```python
from build123d import *
from build123d.topology import SkipClean

# Parameters (mm, degrees)
SKETCH2_R               = 120
BOSS_EXTRUDE2_DEPTH     = 85
SKETCH3_R               = 116
CUT_EXTRUDE1_DEPTH      = 82
CUT_EXTRUDE5_DEPTH      = 2
CUT_EXTRUDE5_DEPTH_BACK = 2
SKETCH8_R               = 75
SKETCH9_R               = 32
CUT_EXTRUDE6_DEPTH      = 5
BOSS_EXTRUDE4_START     = 40
SKETCH12_R              = 32
BOSS_EXTRUDE4_DEPTH     = 40


with BuildPart() as part:
    # Sketch2 → Boss-Extrude2 (new body)
    with BuildSketch(Plane.XY):
        Circle(SKETCH2_R)
    extrude(amount=BOSS_EXTRUDE2_DEPTH)

    # Sketch3 → Cut-Extrude1 (cut)
    with BuildSketch(Plane.XY.offset(85)):
        Circle(SKETCH3_R)
    extrude(amount=-CUT_EXTRUDE1_DEPTH, mode=Mode.SUBTRACT)

    # Sketch8 → Cut-Extrude5 (cut, two sides: drawn at the far end of the back side and taken through both)
    with BuildSketch(Plane.XY.offset(3).offset(-CUT_EXTRUDE5_DEPTH_BACK)):
        Circle(SKETCH8_R)
    extrude(amount=CUT_EXTRUDE5_DEPTH + CUT_EXTRUDE5_DEPTH_BACK, mode=Mode.SUBTRACT)

    # Sketch9 → Cut-Extrude6 (cut)
    with BuildSketch(Plane.XY.offset(1)):
        Circle(SKETCH9_R)
    extrude(amount=-CUT_EXTRUDE6_DEPTH, mode=Mode.SUBTRACT)

    # Sketch12 → Boss-Extrude4 (add)
    # profile 1 of 2: a face of its own
    with SkipClean():  # the faces are left unmerged after this step: merging them gives an invalid solid
        with BuildSketch(Plane(origin=(0, 0, 0), x_dir=(-1, 0, 0), z_dir=(0, 0, -1)).offset(BOSS_EXTRUDE4_START)):
            with BuildLine():
                ThreePointArc((120, 0), (0, 120), (-120, 0))
                Line((-120, 0), (-118.831087629, -16.70845932))
                ThreePointArc((-118.831087629, -16.70845932), (-3.111785776, -119.959646504), (117.805011812, -22.84686394))
                Line((117.805011812, -22.84686394), (120, 0))
            make_face()
            with Locations(Location((0, 0, 0), (0, 0, 180))):
                Circle(SKETCH12_R, mode=Mode.SUBTRACT)
        # profile 2 of 2: a face of its own
        with BuildSketch(Plane(origin=(0, 0, 0), x_dir=(-1, 0, 0), z_dir=(0, 0, -1)).offset(BOSS_EXTRUDE4_START)):
            with BuildLine():
                ThreePointArc((117.805011812, -22.84686394), (-3.111785776, -119.959646504), (-118.831087629, -16.70845932))
                Line((-118.831087629, -16.70845932), (-99.063378042, -299.268538041))
                ThreePointArc((-99.063378042, -299.268538041), (-3.575656086, -388.008129656), (91.309922092, -298.624981255))
                Line((91.309922092, -298.624981255), (117.805011812, -22.84686394))
            make_face()
        extrude(amount=-BOSS_EXTRUDE4_DEPTH)


solid = part.part
```
The listing builds one solid part. Answer for the finished solid, in the listing's coordinates (mm). A direction names the side the tool comes from. Give positions to 0.01 mm unless a question says otherwise; leave off trailing zeros. Loops run counter-clockwise (first coordinate to the right, second up) from the corner with the lowest first, then second, coordinate; pieces in that order, holes last. Notation, with made-up numbers: (77.5, -6) - (120.5, -6) arc R21 ccw to (120.5, 25) - close; hole circle Ø7 at (53, 6.5). An arc over 180 degrees is marked (long way). Answer as CSV lines item,"result". Start each with the question number.
Item 1: A cutting plane is placed at A-A on x = -1. Determine the outline of the cut face in (y, z), then the cut area to 3 significant figures.
Item 2: A cutting plane is placed at C-C on x = -60.5. Determine the outline of the cut face in (y, z).
Item 3: For faces 4 (the face through (-63, 98, 85)), 5 (the face through (-2, -76, 3)), determine the directions among +Z, -Z, +X, -X, +Y, -Y from which every point of the face is accessible in a straight line to the end or side of a thin tool.
Item 4: A cutting plane is placed at B-B on y = -64. Determine the outline of the cut face in (x, z), then the cut area to 3 significant figures.
Item 5: Each of these flat-tipped pins is pushed along its axis until it touches: pin 1 (3 mm diameter, centred on x = -74.5, z = 38.5, fed in from -Y); pin 2 (2 mm diameter, centred on x = 5.5, z = -2.5, fed in from +Y); pin 3 (10 mm diameter, centred on y = -244.5, z = 0.5, fed in from +X). Where does it stop, or does it pass through?
Item 6: A cutting plane is placed at D-D on z = 73. Determine the outline of the cut face in (x, y), then the cut area to 3 significant figures.
Item 7: Find the intervals of material crossed by line 1 (Y direction, x = 0, z = -21); line 2 (Z direction, x = -105, y = -45); line 3 (Z direction, x = -11, y = -277), in increasing order. Write a range as from..to.
Item 8: The mould has two halves that part along X. Classify faces 1 (the face through (2, -241, 0)), 2 (the face through (5.585, -387.994, -20.28)), 3 (the face through (-9.764, 74.362, 1.986)): +X half, -X half, draft (parallel to the pull), parting line (faces both ways), or undercut.
Found:
1,outline,"(-387.88, -40) - (-31.98, -40) - (-31.98, 1) - (-74.99, 1) - (-74.99, 3) - (-116, 3) - (-116, 85) - (-120, 85) - (-120, 0) - (-387.88, 0) - close; (31.98, -40) - (120, -40) - (120, 85) - (116, 85) - (116, 3) - (74.99, 3) - (74.99, 1) - (31.98, 1) - close"
1,area,"18,800 mm^2"
2,outline,"(-362.99, -40) - (103.63, -40) - (103.63, 85) - (98.97, 85) - (98.97, 3) - (44.33, 3) - (44.33, 1) - (-44.33, 1) - (-44.33, 3) - (-98.97, 3) - (-98.97, 85) - (-103.63, 85) - (-103.63, 0) - (-362.99, 0) - close"
3,face 4,"+Z, +X, -X, +Y, -Y"
3,face 5,"+Z"
4,outline,"(-113.85, -40) - (115.52, -40) - (115.52, 0) - (101.51, 0) - (101.51, 85) - (96.75, 85) - (96.75, 3) - (39.1, 3) - (39.1, 1) - (-39.1, 1) - (-39.1, 3) - (-96.75, 3) - (-96.75, 85) - (-101.51, 85) - (-101.51, 0) - (-113.85, 0) - close"
4,area,"10,400 mm^2"
5,pin 1,"stops at y = -95.24"
5,pin 2,"stops at y = 119.92"
5,pin 3,"stops at x = 103.24"
6,outline,"circle Ø240 at (0, 0); hole circle Ø232 at (0, 0)"
6,area,"2,970 mm^2"
7,line 1,"y = -387.93..-32, 32..120"
7,line 2,"z = -40..3"
7,line 3,"z = -40..0"
8,face 1,"draft"
8,face 2,"parting line"
8,face 3,"undercut"
